Design review of the part built by this model. Coordinates are the model's own, in mm. Face numbers are marked on the shaded views. Give positions to 0.01 mm unless a question says otherwise; leave off trailing zeros. Loops run counter-clockwise (first coordinate to the right, second up) from the corner with the lowest first, then second, coordinate; pieces in that order, holes last. Notation, with made-up numbers: (69.5, 45) - (79.5, 45) arc R20 cw to (79.5, 64) - close; hole circle Ø10 at (-13.75, -38.75). An arc over 180 degrees is marked (long way). Put each result on its own line as item: value. Start each with the question number.
```python
from build123d import *

# Parameters (mm, degrees)
F0_R     = 47.0125269351
F0_R_2   = 38.3432556573
F1_DEPTH = 101.6
F4_DEPTH = 25.4
F5_DEPTH = 25.4
F6_DEPTH = 25.4


with BuildPart() as f1:
    # F0 (on Top) → F1 (new body)
    with BuildSketch(Plane.XY):
        Circle(F0_R)
        Circle(F0_R_2, mode=Mode.SUBTRACT)
    extrude(amount=F1_DEPTH)

    # F4 (add): a face of the model
    f4_faces = [f1.faces().sort_by_distance(p)[0] for p in [
        (-45.6828118712, 0, 101.6),
    ]]
    extrude(f4_faces, amount=F4_DEPTH)

    # F5 (add): a face of the model
    f5_faces = [f1.faces().sort_by_distance(p)[0] for p in [
        (-45.6828118712, 0, 127),
    ]]
    extrude(f5_faces, amount=F5_DEPTH)

    # F3 (on face) → F6 (join)
    with BuildSketch(Plane.XY.offset(101.6)):
        with BuildLine():
            ThreePointArc((7.9259239137, -46.3395880316), (-0.4478621348, -47.0103936202), (-8.8073480874, -46.180172244))
            Line((-8.8073480874, -46.180172244), (-8.8073480874, -49.2319874465))
            Line((-8.8073480874, -49.2319874465), (7.9259239137, -49.2319874465))
            Line((7.9259239137, -49.2319874465), (7.9259239137, -46.3395880316))
        make_face()
    extrude(amount=F6_DEPTH)


solid = f1.part
```
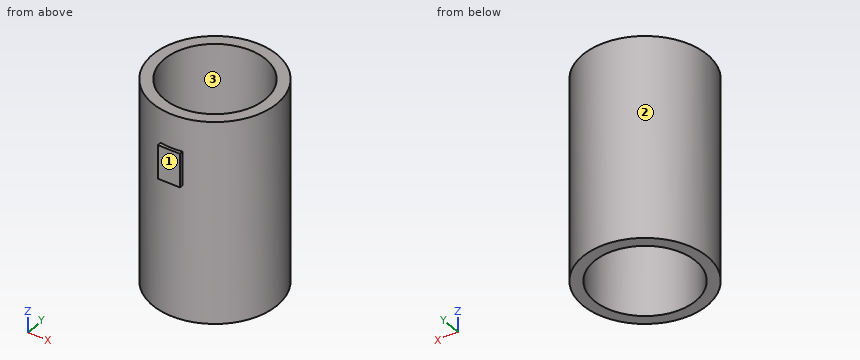
Item 1: For P1, Ø1.5, axis at x = 29, z = 29, coming from the -Y side; P2, Ø2.5, axis at y = -48.5, z = 118, coming from the -X side; P3, Ø1.5, axis at y = 3, z = 29, coming from the -X side, all flat-tipped, find the tip position at first contact; note any pin that passes through.
Item 2: Consider section D-D (x = 14). State the section outline as (y, z) points, plus the area to 3 significant figures.
Item 3: Consider section A-A (x = 0). State the section outline as (y, z) points.
Item 4: Consider section B-B (y = 0). State the section outline as (x, z) points, plus the area to 3 significant figures.
Item 5: Mouldability with a two-part tool opening along Y and no side actions: class the marked faces 1, 2 and 3 as pulls with the +Y half, pulls with the -Y half, needs draft (parallel to the pull), parting line crosses it, or undercut.
Item 6: Consider section C-C (z = 113.5). State the section outline as (x, y) points.
Item 7: For L1, parallel to Y at x = 0, z = 68; L2, parallel to Y at x = -23, z = 11.5; L3, parallel to X at y = -12, z = 74, list the stretches that pass through material, from the lowest coordinate up. Write a range as from..to.
Geometry says:
1. P1: stops at y = -37.58
1. P2: stops at x = -8.81
1. P3: stops at x = -46.96
2. outline: (-44.88, 0) - (-35.7, 0) - (-35.7, 152.4) - (-44.88, 152.4) - close; (35.7, 0) - (44.88, 0) - (44.88, 152.4) - (35.7, 152.4) - close
2. area: 2,800 mm2
3. outline: (-49.23, 101.6) - (-47.01, 101.6) - (-47.01, 0) - (-38.34, 0) - (-38.34, 152.4) - (-47.01, 152.4) - (-47.01, 127) - (-49.23, 127) - close; (38.34, 0) - (47.01, 0) - (47.01, 152.4) - (38.34, 152.4) - close
4. outline: (-47.01, 0) - (-38.34, 0) - (-38.34, 152.4) - (-47.01, 152.4) - close; (38.34, 0) - (47.01, 0) - (47.01, 152.4) - (38.34, 152.4) - close
4. area: 2,640 mm2
5. face 1: pulls with the -Y half
5. face 2: parting line crosses it
5. face 3: undercut
6. outline: (-8.81, -49.23) - (7.93, -49.23) - (7.93, -46.34) arc R47.01 ccw (long way) to (-8.81, -46.18) - close; hole circle Ø76.69 at (0, 0)
7. L1: y = -47.01..-38.34, 38.34..47.01
7. L2: y = -41..-30.68, 30.68..41
7. L3: x = -45.46..-36.42, 36.42..45.46
